Input: part model. Units: mm. Frame: model coordinates. A direction names the side the tool comes from. Give positions to 0.01 mm unless a question says otherwise; leave off trailing zeros. Order: outer loops, then holes, each group sorted by start corner. A loop starts at its lowest first (then second) coordinate and runs counter-clockwise, first axis right, second up.
```python
from build123d import *

# Parameters (mm, degrees)
F0_W      = 25.4
F0_H      = 25.4
F1_DEPTH  = 25.4
F2_W      = 31.493294
F2_H      = 25.251383
F3_DEPTH  = 12.7
F4_R      = 6.077907
F5_DEPTH  = 25.4
F5_FACE_R = 6.077907
F6_DEPTH  = 50.8
F8_DEPTH  = 12.7


with BuildPart() as f1:
    # F0 (on Front) → F1 (new body)
    with BuildSketch(Plane.XZ):
        with Locations((-57.573333, 12.7)):
            Rectangle(F0_W, F0_H)
        with BuildLine():
            ThreePointArc((-44.873333, 25.4), (-57.573333, 38.1), (-70.273333, 25.4))
            Line((-70.273333, 25.4), (-44.873333, 25.4))
        make_face()
    extrude(amount=F1_DEPTH)

    # F2 (on Top) → F3 (join)
    with BuildSketch(Plane.XY):
        with Locations((-29.932818, -12.625692)):
            Rectangle(F2_W, F2_H)
        with BuildLine():
            ThreePointArc((-14.186171, -25.251383), (-1.560479, -12.625691), (-14.186171, 0))
            Line((-14.186171, 0), (-14.186171, -25.251383))
        make_face()
    extrude(amount=F3_DEPTH)

    # F4 (on face) → F5 (join)
    with BuildSketch(Plane.XZ.offset(25.4)):
        with Locations((-57.573333, 25.4)):
            Circle(F4_R)
    extrude(amount=F5_DEPTH)

    # F5_face (on face) → F6 (cut)
    with BuildSketch(Plane(origin=(-57.573333, -50.8, 25.4), x_dir=(1, 0, 0), z_dir=(0, -1, 0))):
        Circle(F5_FACE_R)
    extrude(amount=-F6_DEPTH, mode=Mode.SUBTRACT)

    # F7 (on face) → F8 (cut)
    with BuildSketch(Plane.XY.offset(12.7)):
        with BuildLine():
            ThreePointArc((-14.186171, -19.293193), (-7.660532, -12.767554), (-14.186171, -6.241916))
            Line((-14.186171, -6.241916), (-38.018938, -6.241916))
            ThreePointArc((-38.018938, -6.241916), (-43.983294, -13.03921), (-37.451491, -19.293193))
            Line((-37.451491, -19.293193), (-14.186171, -19.293193))
        make_face()
    extrude(amount=-F8_DEPTH, mode=Mode.SUBTRACT)


solid = f1.part
```
1) Cut plane D-D (z = 17). Return the cut outline in (x, y), then the cut area to 3 significant figures.
2) Cut plane A-A (y = -9.75). Return the cut outline in (x, z), then the cut area to 3 significant figures.
3) Cut plane C-C (z = 21). Return the cut outline in (x, y), then the cut area to 3 significant figures.
4) Reachability of faces 1 (the face through (-58, -25.4, 15)), 2 (the face through (-30, -25.251, 6)), 3 (the face through (-7.662, -12.911, 6.439)), 4 (the face through (-57.294, -12.522, 38.097)), 5 (the face through (-24, -4, 12.7)) from +Z, -Z, +X, -X, +Y, -Y: full face, straight path, thin tool, end or side. Return the list, or none.
5) Pull-direction query (X, two-part tool) for faces 6 (the face through (-51.776, -12.878, 27.226)), 7 (the face through (-1.564, -12.903, 6.261)), 8 (the face through (-43.988, -12.899, 6.439)), 9 (the face through (-70.273, -13, 13)); classes: pulls with the +X half, pulls with the -X half, needs draft (parallel to the pull), parting line crosses it, or undercut.
6) Cut plane B-B (x = -33.5). Return the cut outline in (y, z).
7) First-contact query: P1, Ø12, axis at x = -21, y = -11.5, coming from the +Z side; P2, Ø2, axis at y = -6.5, z = 28.5, coming from the -X side; P3, Ø10, axis at x = -20.5, z = 4.5, coming from the -Y side; P4, Ø4, axis at x = -59, y = -9.5, coming from the -Z side. Flat tips, straight axial feed; report the tip coordinate or a pass-through.
8) Line query: probe 1 along Z at (x, y) = (-26.5, -20.5); probe 2 along X at (y, z) = (-6.25, 17); probe 3 along Z at (x, y) = (-55.5, -19.75). Output: solid intervals per line, ascending.
Geometry says:
1. outline: (-70.27, -25.4) - (-44.87, -25.4) - (-44.87, 0) - (-70.27, 0) - close
1. area: 645 mm2
2. outline: (-70.27, 0) - (-43.26, 0) - (-43.26, 12.7) - (-44.87, 12.7) - (-44.87, 25.4) arc R12.7 ccw to (-70.27, 25.4) - close; (-8.4, 0) - (-1.89, 0) - (-1.89, 12.7) - (-8.4, 12.7) - close; hole circle Ø12.16 at (-57.57, 25.4)
2. area: 886 mm2
3. outline: (-70.27, -25.4) - (-61.77, -25.4) - (-61.77, 0) - (-70.27, 0) - close; (-53.38, -25.4) - (-44.87, -25.4) - (-44.87, 0) - (-53.38, 0) - close
3. area: 432 mm2
4. face 1: +Z, -Z, +X, -X, -Y
4. face 2: +Z, -Z, +X, -Y
4. face 3: +Z, -Z
4. face 4: +Z, +Y, -Y
4. face 5: +Z, +X, +Y, -Y
5. face 6: undercut
5. face 7: pulls with the +X half
5. face 8: undercut
5. face 9: pulls with the -X half
6. outline: (-25.25, 0) - (-19.29, 0) - (-19.29, 12.7) - (-25.25, 12.7) - close; (-6.24, 0) - (0, 0) - (0, 12.7) - (-6.24, 12.7) - close
7. P1: stops at z = 12.7
7. P2: stops at x = -70.1
7. P3: stops at y = -25.25
7. P4: stops at z = 0
8. probe 1: z = 0 to 12.7
8. probe 2: x = -70.27 to -44.87
8. probe 3: z = 0 to 19.69, 31.11 to 37.93
